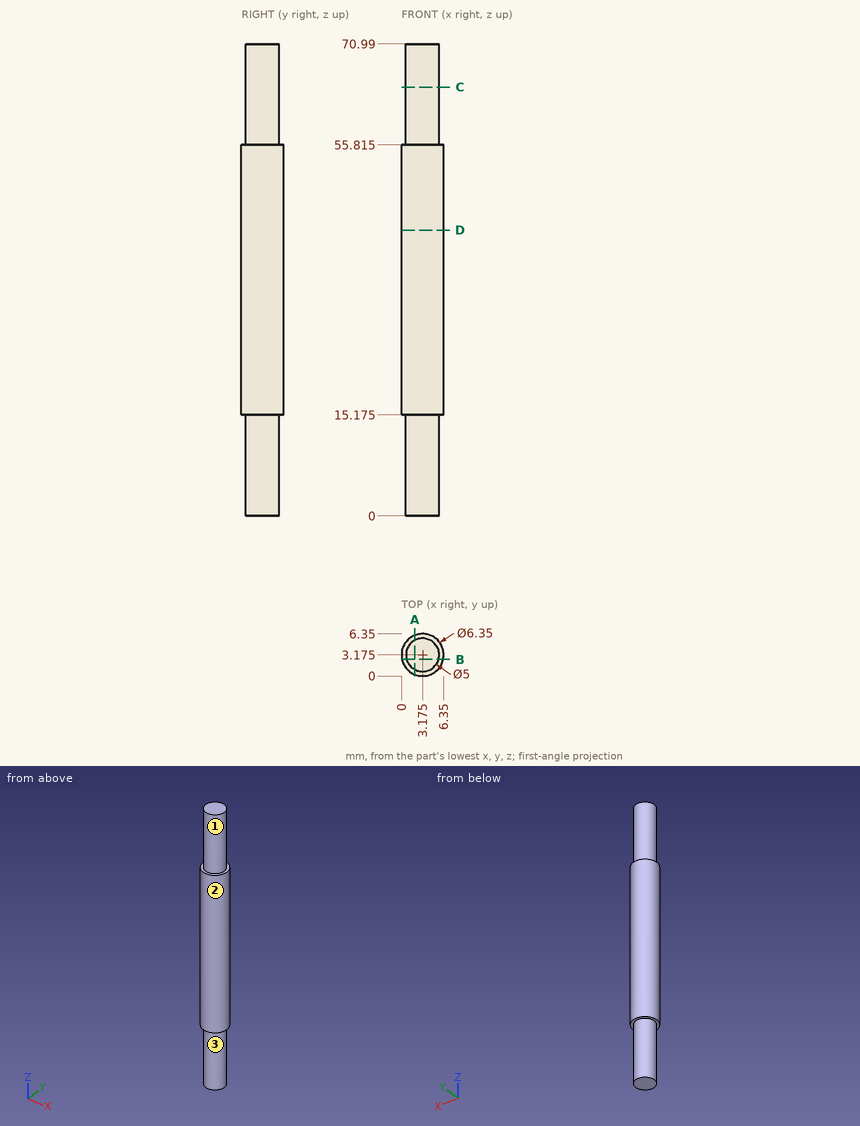
Check sheet for the drawn part. Datum: minimum x, y, z corner. Units: mm. A direction names the side the tool comes from. Give positions to 0.01 mm unless a question says otherwise; leave off trailing zeros. Order: outer loops, then holes, each group sorted by start corner. A loop starts at its lowest first (then second) coordinate and runs counter-clockwise, first axis right, second up. Notation, with made-up numbers: (41, 41) - (85, 41) arc R17 cw to (85, 57) - close; hole circle Ø1 at (-10, 23). An arc over 180 degrees is marked (long way). Answer in a Markdown table with one row per item. Add a question column.
Q1. Cross-section at A-A, the plane x = 2. Enter the section's corners in (y, z) (1 decimal).
Q2. Tool access check on the marked faces 1, 2 and 3. Record the directions out of +Z, -Z, +X, -X, +Y, -Y that give a thin tool (end or side, any length) a straight path to the whole face; none if there is none.
Q3. Material ranges on probe 1 along Z at (x, y) = (4.75, 1) (3 decimals); probe 2 along X at (y, z) = (3.25, 40); probe 3 along X at (y, z) = (2.5, 41.5), recorded low to high. Write a range as from..to.
Q4. Gauge pin test, flat ends, axial feed: pin 1 (1 mm diameter, centred on x = 5.5, y = 5, fed in from +Z); pin 2 (1.5 mm diameter, centred on x = 5, z = 20, fed in from +Y). Record the tip position at first contact, or that the pin passes through.
Q5. Cross-section at B-B, the plane y = 2.5. Enter the section's corners in (x, z) (1 decimal).
Q6. Cross-section at C-C, the plane z = 64.5. Enter the section's corners in (x, y) (3 decimals), then the cut area to 3 significant figures.
Q7. Cross-section at D-D, the plane z = 43. Enter the section's corners in (x, y) (3 decimals), then the cut area to 3 significant figures.
Check values:
| question | item | result |
|---|---|---|
| 1 | outline | (0.2, 15.2) - (1, 15.2) - (1, 0) - (5.4, 0) - (5.4, 15.2) - (6.1, 15.2) - (6.1, 55.8) - (5.4, 55.8) - (5.4, 71) - (1, 71) - (1, 55.8) - (0.2, 55.8) - close |
| 2 | face 1 | +Z |
| 2 | face 2 | +Z, -Z |
| 2 | face 3 | -Z |
| 3 | probe 1 | z = 15.175..55.815 |
| 3 | probe 2 | x = 0..6.35 |
| 3 | probe 3 | x = 0.07..6.28 |
| 4 | pin 1 | stops at z = 70.99 |
| 4 | pin 2 | stops at y = 6.16 |
| 5 | outline | (0.1, 15.2) - (0.8, 15.2) - (0.8, 0) - (5.6, 0) - (5.6, 15.2) - (6.3, 15.2) - (6.3, 55.8) - (5.6, 55.8) - (5.6, 71) - (0.8, 71) - (0.8, 55.8) - (0.1, 55.8) - close |
| 6 | outline | circle Ø5 at (3.175, 3.175) |
| 6 | area | 19.6 mm^2 |
| 7 | outline | circle Ø6.35 at (3.175, 3.175) |
| 7 | area | 31.7 mm^2 |
